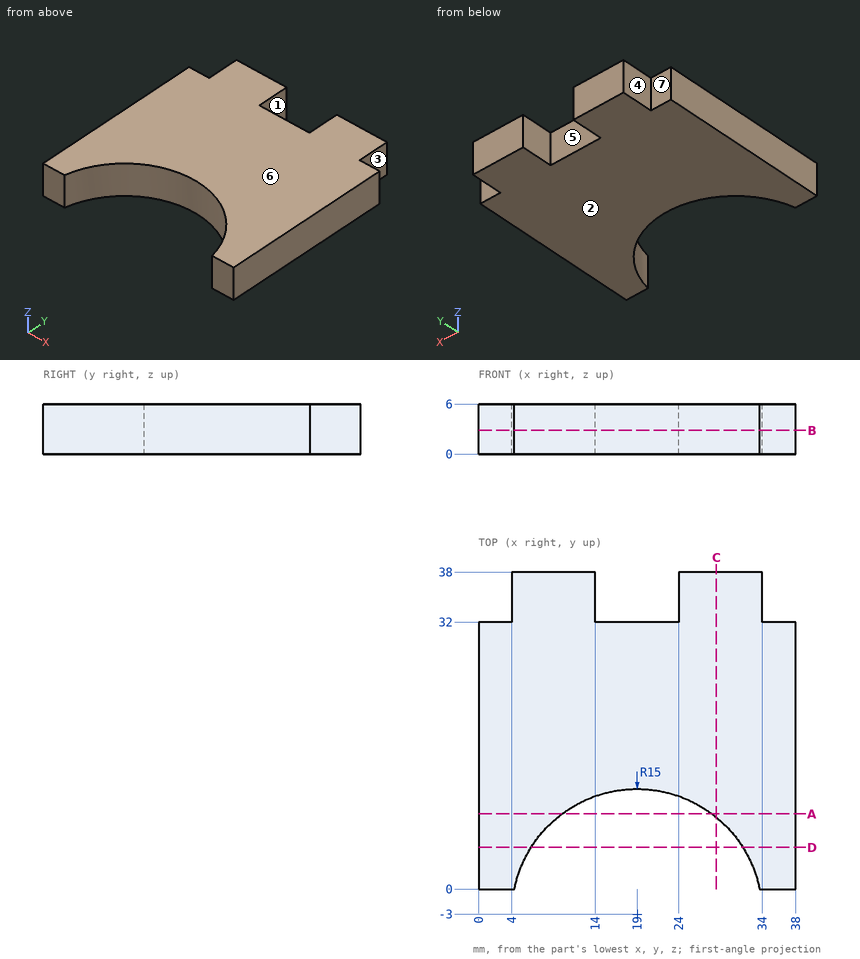
Print and shaded views of the part. All mm, measured from the part's lowest x, y and z. A direction names the side the tool comes from. Round coordinates to 2 decimals unless told otherwise and drop trailing zeros. Order: outer loops, then holes, each group sorted by start corner. A loop starts at its lowest first (then second) coordinate and runs counter-clockwise, first axis right, second up. Notation, with made-up numbers: (3.5, -17) - (7.5, -17) arc R22 cw to (7.5, -5) - close; hole circle Ø7 at (63, 17.5). An arc over 180 degrees is marked (long way). Use a Markdown table: item, result.
1) Flat gauge pins, fed straight in: pin 1 Ø3 at (y, z) = (36, 2) entering from -X; pin 2 Ø2 at (x, z) = (17.5, 4.5) entering from +Y; pin 3 Ø3 at (y, z) = (36.5, 3) entering from +X. Where does each tip first touch, or does it go through?
Recorded:
| item | result |
|---|---|
| pin 1 | stops at x = 4 |
| pin 2 | stops at y = 32 |
| pin 3 | stops at x = 34 |
2) Tool access for the marked faces 5, 6 and 7: list every direction of +Z, -Z, +X, -X, +Y, -Y with a clear straight run to the whole face (end or side of a thin tool).
Recorded:
| item | result |
|---|---|
| face 5 | +Z, -Z, +Y |
| face 6 | +Z, +X, -X, +Y, -Y |
| face 7 | +Z, -Z, -X, +Y |
3) Saw through at B-B on z = 2.85. Write the cut outline in (x, y).
Recorded:
| item | result |
|---|---|
| outline | (0, 0) - (4.3, 0) arc R15 cw to (33.7, 0) - (38, 0) - (38, 32) - (34, 32) - (34, 38) - (24, 38) - (24, 32) - (14, 32) - (14, 38) - (4, 38) - (4, 32) - (0, 32) - close |
4) Saw through at A-A on y = 9. Write the cut outline in (x, z), and give its area (3 significant figures).
Recorded:
| item | result |
|---|---|
| outline | (0, 0) - (10, 0) - (10, 6) - (0, 6) - close; (28, 0) - (38, 0) - (38, 6) - (28, 6) - close |
| area | 120 mm² |
5) Saw through at D-D on y = 5. Write the cut outline in (x, z).
Recorded:
| item | result |
|---|---|
| outline | (0, 0) - (6.31, 0) - (6.31, 6) - (0, 6) - close; (31.69, 0) - (38, 0) - (38, 6) - (31.69, 6) - close |
6) Wall check: L1, parallel to X at y = 33, z = 4.2; L2, parallel to X at y = 7.5, z = 3.85; L3, parallel to Y at x = 2.5, z = 5.1. Give the ranges that are in metal, low to high.
Recorded:
| item | result |
|---|---|
| L1 | x = 4 to 14, 24 to 34 |
| L2 | x = 0 to 8.29, 29.71 to 38 |
| L3 | y = 0 to 32 |
7) Saw through at C-C on x = 28.5. Write the cut outline in (y, z).
Recorded:
| item | result |
|---|---|
| outline | (8.61, 0) - (38, 0) - (38, 6) - (8.61, 6) - close |
8) Pull direction X, two halves, no side cores. Call the marked faces 1, 2, 3 and 4: pulls with the +X half, pulls with the -X half, needs draft (parallel to the pull), parting line crosses it, or undercut.
Recorded:
| item | result |
|---|---|
| face 1 | undercut |
| face 2 | needs draft |
| face 3 | pulls with the +X half |
| face 4 | pulls with the -X half |
